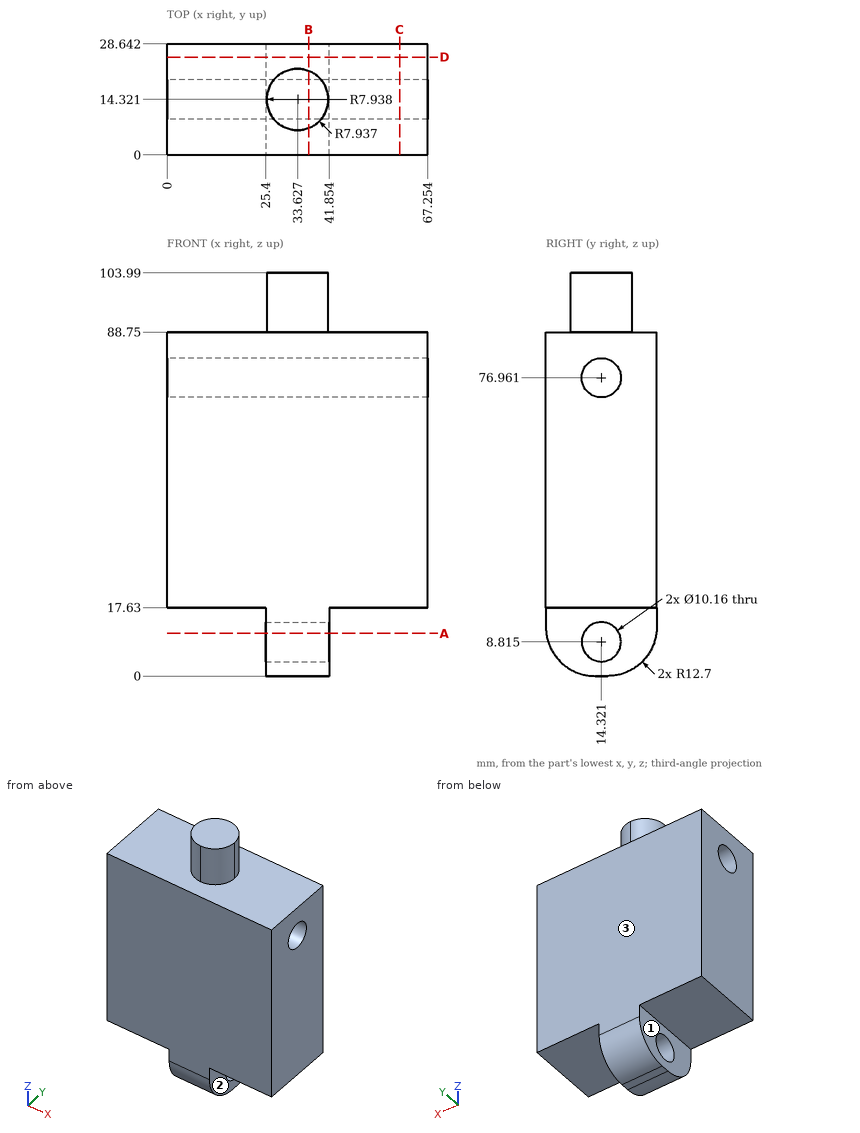
Verification items for this drawing (mm, ordinates from the low corner). A direction names the side the tool comes from. Coordinates: 2 decimals unless noted, no trailing zeros. Loops run counter-clockwise (first coordinate to the right, second up) from the corner with the lowest first, then second, coordinate; pieces in that order, holes last. Notation, with made-up numbers: (-6.75, 25) - (2.25, 25) arc R22 ccw to (2.25, 53) - close; hole circle Ø5 at (48, 57). An arc over 180 degrees is marked (long way). One line per item, written item: value. Start each with the question number.
(1) Material ranges on line 1 (Z direction, x = 37, y = 15.75) (1 decimal); line 2 (Z direction, x = 25.5, y = 12.5); line 3 (Z direction, x = 42, y = 21), recorded low to high. Write a range as [from, to].
(2) Cross-section at D-D on y = 25.25. Enter the section's corners in (x, z), plus the area to 3 significant figures.
(3) Cross-section at B-B on x = 36.5. Count the separate pieces of the cut face and the enclosed holes in it, plus the area to 3 significant figures.
(4) Tool access check on the marked faces 1, 2 and 3. Record the directions out of +Z, -Z, +X, -X, +Y, -Y that give a thin tool (end or side, any length) a straight path to the whole face; none if there is none.
(5) Cross-section at C-C on x = 60. Enter the section's corners in (y, z).
(6) Depth check by flat-ended pin: P1, Ø6, axis at x = 11, y = 6, coming from the -Z side; P2, Ø14, axis at y = 15.5, z = 5.5, coming from the -X side; P3, Ø5, axis at y = 19.5, z = 15.5, coming from the +X side; P4, Ø14, axis at y = 8.5, z = 7.5, coming from the +X side. Enter the tip coordinate at first touch or a pass-through.
(7) Cross-section at A-A on z = 11. Enter the section's corners in (x, y) (1 decimal).
Results below:
1. line 1: z = [0, 3.9], [13.7, 72.1], [81.8, 104]
1. line 2: z = [0, 4.07], [13.56, 72.22], [81.7, 88.75]
1. line 3: z = [17.63, 88.75]
2. outline: (0, 17.63) - (25.4, 17.63) - (25.4, 4.06) - (41.85, 4.06) - (41.85, 17.63) - (67.25, 17.63) - (67.25, 88.75) - (0, 88.75) - close
2. area: 5,010 mm2
3. separate pieces: 1
3. enclosed holes: 2
3. area: 2,540 mm2
4. face 1: -Z, -X, +Y, -Y
4. face 2: -Z, +X, +Y, -Y
4. face 3: +Z, -Z, +X, -X, +Y
5. outline: (0, 17.63) - (28.64, 17.63) - (28.64, 88.75) - (0, 88.75) - close; hole circle Ø10.16 at (14.32, 76.96)
6. P1: stops at z = 17.63
6. P2: stops at x = 25.4
6. P3: stops at x = 67.25
6. P4: stops at x = 41.85
7. outline: (25.4, 0.1) - (41.9, 0.1) - (41.9, 9.7) - (25.4, 9.7) - close; (25.4, 18.9) - (41.9, 18.9) - (41.9, 28.5) - (25.4, 28.5) - close
